Answer from the drawing. Dimensions are ordinates in mm from the lowest x, y and z of the part. Coordinates: 2 decimals unless noted, no trailing zeros. Write each loop counter-clockwise with the first axis right and the second up, starting at its lowest first coordinate (ties: lowest second). Pieces come first, ordered by that corner, then holes.
(1) Section C-C on z = 4 is taken. Write down the section's boundary in (x, y).
(2) Section D-D on x = 74 is taken. Write down the section's boundary in (y, z).
(3) Given pin 1 (1.2 mm diameter, centred on x = 46, y = 86.5, fed in from -Z); pin 2 (4.5 mm diameter, centred on x = 83.35, y = 30.5, fed in from -Z); pin 3 (4 mm diameter, centred on y = 57.5, z = 2, fed in from -X); pin 4 (1 mm diameter, centred on y = 59.5, z = 5, fed in from +X), each flat-ended and moving along its own axis, determine where each tip first touches the part or whether it passes through.
(4) Section A-A on x = 45 is taken. Write down the section's boundary in (y, z), then the cut area to 3 significant figures.
(5) Find the intervals of material crossed by probe 1 along Y at (x, z) = (45, 0.5); probe 2 along Y at (x, z) = (57, 4.75); probe 3 along X at (y, z) = (67, 6.75) (1 decimal), in increasing order.
(6) Section B-B on y = 86 is taken. Write down the section's boundary in (x, z), then the cut area to 3 significant figures.
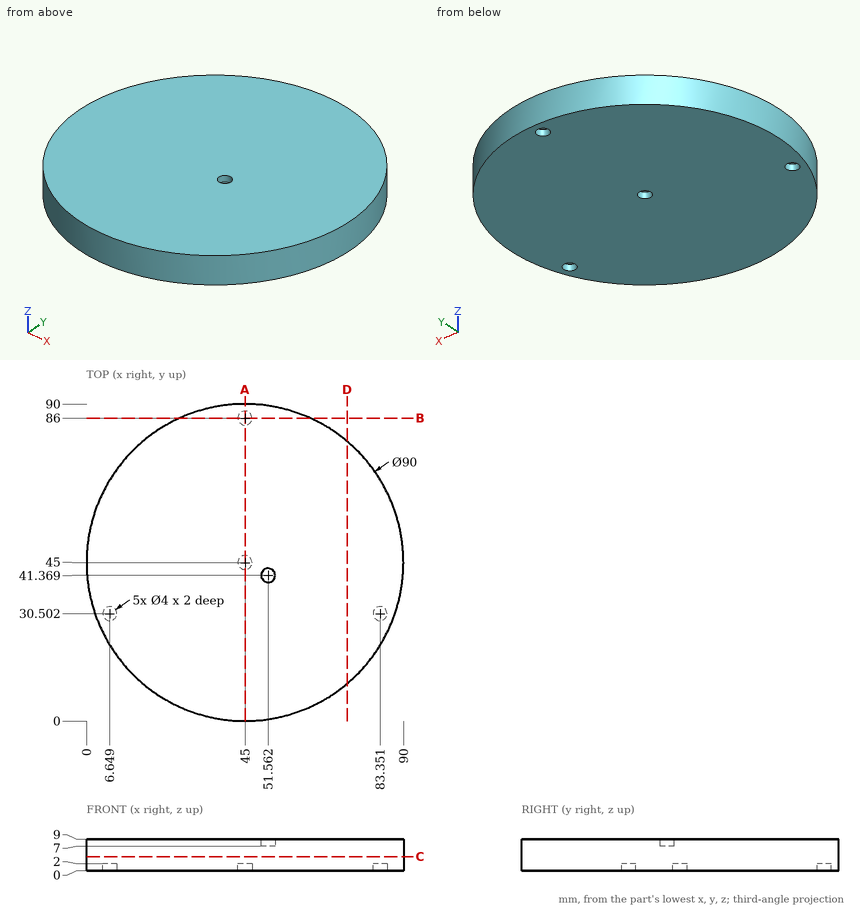
Response:
1. outline: circle Ø90 at (45, 45)
2. outline: (10.59, 0) - (79.41, 0) - (79.41, 9) - (10.59, 9) - close
3. pin 1: stops at z = 2
3. pin 2: stops at z = 0
3. pin 3: stops at x = 1.24
3. pin 4: stops at x = 87.77
4. outline: (0, 0) - (43, 0) - (43, 2) - (47, 2) - (47, 0) - (84, 0) - (84, 2) - (88, 2) - (88, 0) - (90, 0) - (90, 9) - (0, 9) - close
4. area: 794 mm2
5. probe 1: y = 0 to 43, 47 to 84, 88 to 90
5. probe 2: y = 1.63 to 88.37
5. probe 3: x = 5.7 to 84.3
6. outline: (26.45, 0) - (43, 0) - (43, 2) - (47, 2) - (47, 0) - (63.55, 0) - (63.55, 9) - (26.45, 9) - close
6. area: 326 mm2
